```python
from build123d import *

# Parameters (mm, degrees)
SKETCH2_W           = 20
SKETCH2_H           = 5
BOSS_EXTRUDE1_DEPTH = 10
SKETCH5_W           = 5
SKETCH5_H           = 5
BOSS_EXTRUDE2_DEPTH = 100
SKETCH6_W           = 5
SKETCH6_H           = 5
BOSS_EXTRUDE3_DEPTH = 85


with BuildPart() as part:
    # Sketch2 → Boss-Extrude1 (new body)
    with BuildSketch(Plane(origin=(0, 0, 0), x_dir=(1, 0, 0), z_dir=(0, 1, 0))):
        Rectangle(SKETCH2_W, SKETCH2_H)
    extrude(amount=BOSS_EXTRUDE1_DEPTH)

    # Sketch5 → Boss-Extrude2 (add)
    with BuildSketch(Plane(origin=(0, 0, 0), x_dir=(1, 0, 0), z_dir=(0, 1, 0))):
        with Locations((-7.5, 0)):
            Rectangle(SKETCH5_W, SKETCH5_H)
    extrude(amount=-BOSS_EXTRUDE2_DEPTH)

    # Sketch6 → Boss-Extrude3 (add)
    with BuildSketch(Plane.XZ):
        with Locations((7.5, 0)):
            Rectangle(SKETCH6_W, SKETCH6_H)
    extrude(amount=BOSS_EXTRUDE3_DEPTH)


solid = part.part
```
Input: part model. Units: mm. Frame: model coordinates. A direction names the side the tool comes from. Give positions to 0.01 mm unless a question says otherwise; leave off trailing zeros. Order: outer loops, then holes, each group sorted by start corner. A loop starts at its lowest first (then second) coordinate and runs counter-clockwise, first axis right, second up. Notation, with made-up numbers: M 50,20.5 L 66,20.5 A18 ccw 66,50.5 Z; hole C 69,76.25 d8. An arc over 180 degrees is marked long. One line per question, with ' | ' between items. Start each with the question number.
1. Pull-direction query (X, two-part tool) for faces 4 (the face through (-10, -44, 0)), 5 (the face through (10, -37, 0)), 6 (the face through (-8, -100, 0)), 7 (the face through (0, 0, 0)); classes: released by +X, released by -X, zero draft, split by the parting line, or undercut.
2. First-contact query: pin 1 Ø1.5 at (x, z) = (1, 1) entering from -Y. Flat tip, straight axial feed; report the tip coordinate or a pass-through.
3. Material intervals for probe 1 along X at (y, z) = (-4, 1); probe 2 along Y at (x, z) = (-4.75, 0.1); probe 3 along Y at (x, z) = (5.25, -0.2), sorted ascending. Write a range as [from, to].
4. Access query for faces 1 (the face through (5, -42, 0)), 2 (the face through (7, -85, 0)), 3 (the face through (-7, -32, -2.5)). Directions: +Z, -Z, +X, -X, +Y, -Y. A direction counts if a zero-diameter tool reaches every point of the face in a straight line with its end or side. Return the directions, or none.
5. Section query B-B (z = 0.8). Return the cut outline in (x, y), and give its area (4 significant figures).
6. Section query D-D (x = 8.75). Return the cut outline in (y, z), and give its area (3 significant figures).
7. Section query A-A (y = -49). Return the cut outline in (x, z), and give its area (3 significant figures).
8. Section query C-C (x = -1.5). Return the cut outline in (y, z).
Here are the results:
1) face 4: released by -X | face 5: released by +X | face 6: zero draft | face 7: undercut
2) pin 1: y = 0
3) probe 1: [-10, -5], [5, 10] | probe 2: [0, 10] | probe 3: [-85, 10]
4) face 1: +Z, -Z, -Y | face 2: +Z, -Z, +X, -Y | face 3: -Z, +X, -X, +Y, -Y
5) outline: M -10,-100 L -5,-100 L -5,0 L 5,0 L 5,-85 L 10,-85 L 10,10 L -10,10 Z | area: 1,125 mm²
6) outline: M -85,-2.5 L 10,-2.5 L 10,2.5 L -85,2.5 Z | area: 475 mm²
7) outline: M -10,-2.5 L -5,-2.5 L -5,2.5 L -10,2.5 Z; M 5,-2.5 L 10,-2.5 L 10,2.5 L 5,2.5 Z | area: 50.0 mm²
8) outline: M 0,-2.5 L 10,-2.5 L 10,2.5 L 0,2.5 Z
